Here's how the part is built. I have some questions about the finished solid (model axes, mm). A direction names the side the tool comes from. Give positions to 0.01 mm unless a question says otherwise; leave off trailing zeros. Write each loop counter-clockwise with the first axis right and the second up, starting at its lowest first coordinate (ties: lowest second). Pieces come first, ordered by that corner, then holes. Notation, with made-up numbers: (32, 38) -> (68, 38) arc R23 ccw to (68, 57) -> close; hole circle Ø1 at (-39.5, 8). An arc over 180 degrees is marked (long way). Return JSON: item names as keys, results as strings.
from build123d import *

# Parameters (mm, degrees)
F0_W     = 26.924
F0_H     = 2.54
F1_DEPTH = 2.54
F2_W     = 29.464
F2_H     = 13.97
F3_DEPTH = 0.762
F4_W     = 29.464
F4_H     = 0.127
F5_DEPTH = 0.254


with BuildPart() as f1:
    # F0 (on Top) → F1 (new body)
    with BuildSketch(Plane.XY):
        with Locations((0, -1.27)):
            Rectangle(F0_W, F0_H)
    extrude(amount=F1_DEPTH)

    # F2 (on Top) → F3 (join)
    with BuildSketch(Plane.XY):
        with Locations((0, -6.985)):
            Rectangle(F2_W, F2_H)
    extrude(amount=-F3_DEPTH)

    # F4 (on face) → F5 (cut)
    with BuildSketch(Plane.XY):
        with Locations((0, -12.6365)):
            Rectangle(F4_W, F4_H)
        with Locations((0, -11.2395)):
            Rectangle(F4_W, F4_H)
        with Locations((0, -9.8425)):
            Rectangle(F4_W, F4_H)
        with Locations((0, -8.4455)):
            Rectangle(F4_W, F4_H)
        with Locations((0, -7.0485)):
            Rectangle(F4_W, F4_H)
        with Locations((0, -5.6515)):
            Rectangle(F4_W, F4_H)
        with Locations((0, -4.2545)):
            Rectangle(F4_W, F4_H)
        with Locations((0, -2.8575)):
            Rectangle(F4_W, F4_H)
        with Locations((0, -1.4605)):
            Rectangle(F4_W, F4_H)
    extrude(amount=-F5_DEPTH, mode=Mode.SUBTRACT)


solid = f1.part
1. For pin 1 Ø1 at (x, y) = (-4, -3.5) entering from +Z, with a flat end and sliding along its axis, tell me the tip position at first contact or that it passes through.
Taken from the geometry:
{"pin 1": "stops at z = 0"}
2. Suppose I cut it at B-B, the plane z = 1.4. List the corners of the cut face in (x, y) for me.
Taken from the geometry:
{"outline": "(-13.46, -2.54) -> (13.46, -2.54) -> (13.46, 0) -> (-13.46, 0) -> close"}
3. Which directions (+Z, -Z, +X, -X, +Y, -Y) give clear straight access to the entire face, cutting with the end or side of a thin tool? Please do faces 1 (the face through (0, -1, 2.54)), 2 (the face through (14, -1, 0)), 3 (the face through (0, 0, 1)), 4 (the face through (-14, -1, 0)), 5 (the face through (0, -6, 0)).
Taken from the geometry:
{"face 1": "+Z, +X, -X, +Y, -Y", "face 2": "+Z, +X, +Y, -Y", "face 3": "+Z, -Z, +X, -X, +Y", "face 4": "+Z, -X, +Y, -Y", "face 5": "+Z, +X, -X, -Y"}
4. Suppose I cut it at A-A, the plane y = -0.75. List the corners of the cut face in (x, z) for me.
Taken from the geometry:
{"outline": "(-14.73, -0.76) -> (14.73, -0.76) -> (14.73, 0) -> (13.46, 0) -> (13.46, 2.54) -> (-13.46, 2.54) -> (-13.46, 0) -> (-14.73, 0) -> close"}
5. Suppose I cut it at C-C, the plane y = -8. List the corners of the cut face in (x, z) for me, and give its area (3 significant figures).
Taken from the geometry:
{"outline": "(-14.73, -0.76) -> (14.73, -0.76) -> (14.73, 0) -> (-14.73, 0) -> close", "area": "22.5 mm²"}
6. If I drill on line 1 (Y direction, x = 10.75, z = 1.15); line 2 (Z direction, x = 5.75, y = -13.5); line 3 (X direction, y = -0.75, z = 0.7), over which ranges is the centre line in solid material (lowest first)? Write a range as [from, to].
Taken from the geometry:
{"line 1": "y = [-2.54, 0]", "line 2": "z = [-0.76, 0]", "line 3": "x = [-13.46, 13.46]"}
